The listing builds one solid part. Answer for the finished solid, in the listing's coordinates (mm). A direction names the side the tool comes from. Give positions to 0.01 mm unless a question says otherwise; leave off trailing zeros. Order: outer loops, then holes, each group sorted by start corner. A loop starts at its lowest first (then second) coordinate and runs counter-clockwise, first axis right, second up. Notation, with made-up numbers: (9, 55) - (47, 55) arc R14 ccw to (47, 77) - close; hole circle Ø4 at (55, 56). An arc over 180 degrees is marked (long way). Write each question's results on one line, items separated by ' | '. Start each with the question number.
1. Flat-ended cylindrical pins translate along their axes: pin 1 (6 mm diameter, centred on y = -6.5, z = 12, fed in from -X); pin 2 (3 mm diameter, centred on x = -3.5, z = 45, fed in from +Y); pin 3 (3 mm diameter, centred on x = -5, y = -11, fed in from +Z). Find the tip coordinate at first contact, or state that the pin passes through.
2. Section B-B (z = 0) is taken. Give the vertices of the cut face in (x, y) (3 decimals).
3. Find the intervals of material crossed by L1, parallel to Z at x = -2.75, y = -6.35 (3 decimals); L2, parallel to Z at x = 4.5, y = -8.75; L3, parallel to Y at x = -3.75, z = 2, in increasing order.
4. Section D-D (y = -2.5) is taken. Give the vertices of the cut face in (x, z).
5. Which of the six approach directions +Z, -Z, +X, -X, +Y, -Y give full straight-line access (tool end or side, diameter ignored) to faces 1 (the face through (6.35, -3, -2)), 2 (the face through (-0.62, -1.63, 37.66))?
6. Determine the mould class of faces 3 (the face through (3, -2, 6.35)), 4 (the face through (0, -12.7, 0)), 5 (the face through (-0.09, -3.18, 0.14)) for opening direction Y: released by +Y, released by -Y, zero draft, split by the parting line, or undercut.
from build123d import *

# Parameters (mm, degrees)
F0_W     = 12.7
F0_H     = 12.7
F1_DEPTH = 12.7
F2_R     = 4.7625
F3_DEPTH = 63.5
F4_R     = 3.175
F5_DEPTH = 12.701


with BuildPart() as f1:
    # F0 (on Front) → F1 (new body)
    with BuildSketch(Plane.XZ):
        Rectangle(F0_W, F0_H)
    extrude(amount=F1_DEPTH)

    # F2 (on face) → F3 (join)
    with BuildSketch(Plane.XY.offset(6.35)):
        with Locations((0, -6.35)):
            Circle(F2_R)
    extrude(amount=F3_DEPTH)

    # F4 (on face) → F5 (cut, through all)
    with BuildSketch(Plane(origin=(-6.35, 0, 0), x_dir=(0, -1, 0), z_dir=(-1, 0, 0))):
        with Locations((6.35, 0)):
            Circle(F4_R)
    extrude(amount=-F5_DEPTH, mode=Mode.SUBTRACT)


solid = f1.part
Reported:
1) pin 1: x = -4.76 | pin 2: y = -2.03 | pin 3: z = 6.35
2) outline: (-6.35, -12.7) - (6.35, -12.7) - (6.35, -9.525) - (-6.35, -9.525) - close; (-6.35, -3.175) - (6.35, -3.175) - (6.35, 0) - (-6.35, 0) - close
3) L1: -6.35 to -3.175, 3.175 to 69.85 | L2: -6.35 to -2.08, 2.08 to 6.35 | L3: -12.7 to -8.82, -3.88 to 0
4) outline: (-6.35, -6.35) - (6.35, -6.35) - (6.35, 6.35) - (2.8, 6.35) - (2.8, 69.85) - (-2.8, 69.85) - (-2.8, 6.35) - (-6.35, 6.35) - close
5) face 1: +Z, -Z, +X, +Y, -Y | face 2: +Z
6) face 3: zero draft | face 4: released by -Y | face 5: undercut
